CAD build for the part. Positions are in the model's coordinates, mm. A direction names the side the tool comes from. Round coordinates to 2 decimals unless told otherwise and drop trailing zeros. Write each loop counter-clockwise with the first axis right and the second up, starting at its lowest first coordinate (ties: lowest second). Pieces come first, ordered by that corner, then holes. Notation, with made-up numbers: (58, -36) - (114, -36) arc R23 cw to (114, -17) - close; hole circle Ø11 at (76, -2). An arc over 180 degrees is marked (long way). Put each result on its own line as item: value. Start each with the question number.
Item 1: Mould opens along X. For faces 4 (the flat face through (65.65, -37.79, 0.99)), 5 (the flat face through (27, -28, -7)), 6 (the cylindrical face through (41.197, 10.533, 4.162)) say: released by +X, released by -X, zero draft, split by the parting line, or undercut.
Item 2: Cut at C-C (x = 66.6). Give the cut face in (y, z).
Item 3: Cut at D-D (z = -3.75). Give the cut face in (x, y).
Item 4: 3-axis set-ups, long thin cutter, end or side, ignore diameter. For faces 1 (the cylindrical face through (-27.712, 11.49, 6.409)), 2 (the flat face through (1.05, -37.96, 0.99)), 3 (the cylindrical face through (30.59, -7.023, -3.451)): which of +Z, -Z, +X, -X, +Y, -Y reach the whole face in a straight line?
Item 5: Pin check, flat tips, straight feed: pin 1 Ø2.5 at (x, y) = (33.5, -13) entering from -Z; pin 2 Ø1.6 at (x, z) = (30, 1) entering from +Y; pin 3 Ø1 at (x, y) = (44, 7) entering from -Z; pin 4 Ø3 at (x, z) = (14, -2) entering from -Y. Stop position of each tip, or through.
Item 6: Drill centre lines: line 1 (Y direction, x = 66.6, z = 3.6); line 2 (Y direction, x = 33.3, z = 0.85); line 3 (Y direction, x = 56, z = 10.75). Where is each one in solid material? Low to high. Write a range as from..to.
Item 7: Cut at B-B (y = 0). Give the cut face in (x, z).
Item 8: Cut at A-A (z = 3.75). Give the cut face in (x, y), and give its area (3 significant figures).
```python
from build123d import *

# Parameters (mm, degrees)
SKETCH_1_R          = 30
SKETCH_1_R_2        = 27.5
EXTRUDE_1_DEPTH     = 13
SKETCH_1_R_3        = 29.999999999999996
EXTRUDE_1_2_DEPTH   = 13
EXTRUDE_1_3_DEPTH   = 13
EXTRUDE_2_DEPTH     = 2
SKETCH_3_R          = 1.3999999999999955
CUT_EXTRUDE_5_DEPTH = 132.10250765535577
FILLET_1_R          = 10
SKETCH_5_R          = 12.500000000000002
SKETCH_5_R_2        = 10.5
EXTRUDE_3_DEPTH     = 7
EXTRUDE_4_DEPTH     = 2


with BuildPart() as part:
    # Sketch 1 → Extrude 1 (new body)
    with BuildSketch(Plane.XY):
        with Locations(Location((0, 0, 0), (0, 0, 180))):
            Circle(SKETCH_1_R)
        with Locations(Location((0, 0, 0), (0, 0, 180))):
            Circle(SKETCH_1_R_2, mode=Mode.SUBTRACT)
    extrude(amount=EXTRUDE_1_DEPTH)



with BuildPart() as body_2:
    # Sketch 1 → Extrude 1 2 (new body)
    with BuildSketch(Plane.XY):
        with Locations(Location((66.6, 0, 0), (0, 0, 180))):
            Circle(SKETCH_1_R_3)
        with Locations(Location((66.6, 0, 0), (0, 0, 180))):
            Circle(SKETCH_1_R_2, mode=Mode.SUBTRACT)
    extrude(amount=EXTRUDE_1_2_DEPTH)


with BuildPart() as body_3:
    # Sketch 1 → Extrude 1 3 (new body)
    with BuildSketch(Plane.XY):
        with Locations(Location((33.30000000000001, -57.6772918920436, 0), (0, 0, 180))):
            Circle(SKETCH_1_R_3)
        with Locations(Location((33.30000000000001, -57.6772918920436, 0), (0, 0, 180))):
            Circle(SKETCH_1_R_2, mode=Mode.SUBTRACT)
    extrude(amount=EXTRUDE_1_3_DEPTH)


with BuildPart() as part_1:
    add(part.part)

    add(body_2.part)  # Extrude 2 merges body 2

    add(body_3.part)  # Extrude 2 merges body 3
    # Sketch 2 → Extrude 2 (add)
    with BuildSketch(Plane.XY):
        with BuildLine():
            Line((26.3198925252566, 18.070831312697457), (40.280107474743396, 18.070831312697457))
            ThreePointArc((40.280107474743396, 18.070831312697457), (42.3441853289733, 18.516758123597654), (44.04009212120862, 19.77499826802639))
            ThreePointArc((44.04009212120862, 19.77499826802639), (92.58076211353317, 15), (72.44569692050842, -29.424952464083248))
            ThreePointArc((72.44569692050842, -29.424952464083248), (70.50807559525407, -30.264530756395246), (69.08985272167097, -31.829111208097117))
            Line((69.08985272167097, -31.829111208097117), (62.10974524692759, -43.91901199664395))
            ThreePointArc((62.10974524692759, -43.91901199664395), (61.46389026628078, -45.92951925924603), (61.70560479929982, -48.027337695986766))
            ThreePointArc((61.70560479929982, -48.027337695986766), (33.300000000000004, -87.6772918920436), (4.894395200700185, -48.02733769598677))
            ThreePointArc((4.894395200700185, -48.02733769598677), (5.13610973371921, -45.92951925924604), (4.4902547530724135, -43.91901199664397))
            Line((4.4902547530724135, -43.91901199664397), (-2.489852721670984, -31.829111208097103))
            ThreePointArc((-2.489852721670984, -31.829111208097103), (-3.9080755952540875, -30.264530756395228), (-5.845696920508439, -29.42495246408323))
            ThreePointArc((-5.845696920508439, -29.42495246408323), (-25.980762113533153, 15.000000000000009), (22.55990787879137, 19.77499826802639))
            ThreePointArc((22.55990787879137, 19.77499826802639), (24.25581467102669, 18.516758123597654), (26.3198925252566, 18.070831312697457))
        make_face()
    extrude(amount=EXTRUDE_2_DEPTH)

    # Sketch 3 → Cut-Extrude 5 (cut, through all)
    with BuildSketch(Plane.XY):
        with Locations(Location((33.3, -19.225763964014533, 0), (0, 0, 180))):
            Circle(SKETCH_3_R)
    extrude(amount=CUT_EXTRUDE_5_DEPTH, mode=Mode.SUBTRACT)

    # Fillet 1
    # the kernel refuses this fillet: 10 mm, written as the material it takes off along each edge
    with BuildSketch(Plane(origin=(0, 0, 13), x_dir=(-1, 1.2e-16, 0), z_dir=(1.2e-16, 1, 0))) as fillet_1_piece_1:
        with BuildLine():
            CenterArc((37.5, -6.614378277661482), FILLET_1_R, 138.59037789072914, 41.409622109270856)
            Line((27.5, -6.614378277661482), (27.3, -6.614378277661482))
            Line((27.3, -6.614378277661482), (27.3, 0))
            Line((27.3, 0), (27.5, 0.1999999999999993))
            ThreePointArc((27.5, 0.1999999999999993), (28.75, 0.1999999999999993), (29.85, 0.1322875655532254))
            Line((29.85, 0.1322875655532254), (30, -3.55e-15))
        make_face()
    revolve(axis=Axis((0, 0, 13), (0, 0, 1)), mode=Mode.SUBTRACT)
    with BuildSketch(Plane(origin=(66.6, 0, 13), x_dir=(-1, 1.2e-16, 0), z_dir=(1.2e-16, 1, 0))) as fillet_1_piece_2:
        with BuildLine():
            CenterArc((37.5, -6.614378277661482), FILLET_1_R, 138.59037789072914, 41.409622109270856)
            Line((27.5, -6.614378277661482), (27.299999999999997, -6.614378277661482))
            Line((27.299999999999997, -6.614378277661482), (27.299999999999997, 0))
            Line((27.299999999999997, 0), (27.5, 0.1999999999999993))
            ThreePointArc((27.5, 0.1999999999999993), (28.75, 0.1999999999999993), (29.85, 0.1322875655532254))
            Line((29.85, 0.1322875655532254), (30, -3.55e-15))
        make_face()
    revolve(axis=Axis((66.6, 0, 13), (0, 0, 1)), mode=Mode.SUBTRACT)
    with BuildSketch(Plane(origin=(33.30000000000001, -57.6772918920436, 13), x_dir=(-1, 0, 0), z_dir=(0, 1, 0))) as fillet_1_piece_3:
        with BuildLine():
            CenterArc((37.5, -6.614378277661478), FILLET_1_R, 138.59037789072914, 41.409622109270856)
            Line((27.5, -6.614378277661478), (27.3, -6.614378277661478))
            Line((27.3, -6.614378277661478), (27.3, 0))
            Line((27.3, 0), (27.5, 0.1999999999999993))
            ThreePointArc((27.5, 0.1999999999999993), (28.75, 0.1999999999999993), (29.849999999999998, 0.1322875655532254))
            Line((29.849999999999998, 0.1322875655532254), (30, -3.55e-15))
        make_face()
    revolve(axis=Axis((33.30000000000001, -57.6772918920436, 13), (0, 0, 1)), mode=Mode.SUBTRACT)

    # Sketch 5 → Extrude 3 (add)
    with BuildSketch(Plane(origin=(0, 0, 0), x_dir=(-1, 0, 0), z_dir=(0, 0, -1))):
        with Locations(Location((-33.3, -19.225763964014533, 0), (0, 0, 180))):
            Circle(SKETCH_5_R)
        with Locations((-33.3, -19.225763964014533)):
            Circle(SKETCH_5_R_2, mode=Mode.SUBTRACT)
    extrude(amount=EXTRUDE_3_DEPTH)

    # Sketch 6 → Extrude 4 (add)
    with BuildSketch(Plane(origin=(0, 0, 0), x_dir=(-1, 0, 0), z_dir=(0, 0, -1))):
        with BuildLine():
            Line((-34.90331925395002, -16.05845163809636), (-43.51884380379272, -16.812212366536837))
            ThreePointArc((-43.51884380379272, -16.812212366536837), (-33.3, -8.725763964014526), (-23.08115619620727, -16.812212366536837))
            Line((-23.08115619620727, -16.812212366536837), (-31.69668074604997, -16.05845163809636))
            ThreePointArc((-31.69668074604997, -16.05845163809636), (-33.3, -15.675763964014527), (-34.90331925395002, -16.05845163809636))
        make_face()
        with BuildLine():
            Line((-34.90331925395002, -22.3930762899327), (-43.51884380379272, -21.63931556149223))
            ThreePointArc((-43.51884380379272, -21.63931556149223), (-33.3, -29.725763964014536), (-23.08115619620727, -21.63931556149223))
            Line((-23.08115619620727, -21.63931556149223), (-31.69668074604997, -22.3930762899327))
            ThreePointArc((-31.69668074604997, -22.3930762899327), (-33.3, -22.775763964014537), (-34.90331925395002, -22.3930762899327))
        make_face()
    extrude(amount=EXTRUDE_4_DEPTH)


solid = part_1.part
```
Output values:
1. face 4: released by +X
1. face 5: zero draft
1. face 6: undercut
2. outline: (-36.14, 0) - (30, 0) - (30, 13) arc R10 ccw to (27.5, 6.39) - (27.5, 2) - (-27.5, 2) - (-27.5, 6.39) arc R10 ccw to (-30, 13) - (-30, 2) - (-36.14, 2) - close
3. outline: circle Ø25 at (33.3, -19.23); hole circle Ø21 at (33.3, -19.23)
4. face 1: +Z
4. face 2: +Z, -Z, -X
4. face 3: -Z
5. pin 1: z = -2
5. pin 2: y = 18.07
5. pin 3: z = 0
5. pin 4: through
6. line 1: -30..-27.5, 27.5..30
6. line 2: -87.68..-20.63, -17.83..18.07
6. line 3: -77.29..-74.91, -40.44..-38.06, -28.06..-26.46, 26.46..28.06
7. outline: (-30, 0) - (96.6, 0) - (96.6, 13) arc R10 ccw to (94.1, 6.39) - (94.1, 2) - (39.1, 2) - (39.1, 6.39) arc R10 ccw to (36.6, 13) - (36.6, 2) - (30, 2) - (30, 13) arc R10 ccw to (27.5, 6.39) - (27.5, 2) - (-27.5, 2) - (-27.5, 6.39) arc R10 ccw to (-30, 13) - close
8. outline: circle Ø60 at (0, 0); circle Ø60 at (33.3, -57.68); circle Ø60 at (66.6, 0); hole circle Ø55 at (0, 0); hole circle Ø55 at (33.3, -57.68); hole circle Ø55 at (66.6, 0)
8. area: 1,350 mm2
